from build123d import *

# Parameters (mm, degrees)
F1_DEPTH = 30.1625
F2_R     = 3.175
F3_DEPTH = 19.051
F4_R     = 3.175
F5_DEPTH = 19.051


with BuildPart() as f1:
    # F0 (on Front) → F1 (new body)
    with BuildSketch(Plane.XZ):
        with BuildLine():
            ThreePointArc((9.525, 7.9375), (9.060032, 9.060032), (7.9375, 9.525))
            Line((7.9375, 9.525), (-7.9375, 9.525))
            ThreePointArc((-7.9375, 9.525), (-9.060032, 9.060032), (-9.525, 7.9375))
            Line((-9.525, 7.9375), (-9.525, -7.9375))
            ThreePointArc((-9.525, -7.9375), (-9.060032, -9.060032), (-7.9375, -9.525))
            Line((-7.9375, -9.525), (7.9375, -9.525))
            ThreePointArc((7.9375, -9.525), (9.060032, -9.060032), (9.525, -7.9375))
            Line((9.525, -7.9375), (9.525, 7.9375))
        make_face()
    extrude(amount=F1_DEPTH)

    # F2 (on face) → F3 (cut, through all)
    with BuildSketch(Plane.XY.offset(9.525)):
        with Locations((0, -23.8125)):
            Circle(F2_R)
    extrude(amount=-F3_DEPTH, mode=Mode.SUBTRACT)

    # F4 (on face) → F5 (cut, through all)
    with BuildSketch(Plane(origin=(-9.525, 0, 0), x_dir=(0, -1, 0), z_dir=(-1, 0, 0))):
        with Locations((6.35, 0)):
            Circle(F4_R)
    extrude(amount=-F5_DEPTH, mode=Mode.SUBTRACT)


solid = f1.part
Geometry: final body of the model. Coordinates: model frame, mm. Coordinates: 2 decimals unless noted, no trailing zeros. Order: outer loops, then holes, each group sorted by start corner. A loop starts at its lowest first (then second) coordinate and runs counter-clockwise, first axis right, second up.
(1) Draft query along X for faces 1 (the face through (-9.05, -14.87, 9.07)), 2 (the face through (1.465, -26.629, 0.133)), 3 (the face through (9.525, -15, 0)). Return one class per face: pulls with the +X half, pulls with the -X half, needs draft (parallel to the pull), parting line crosses it, or undercut.
(2) Section query B-B (x = 0). State how many separate pieces and enclosed holes the cut face has, plus the area to 3 significant figures.
(3) Section query A-A (y = -6.35). Return the cut outline in (x, z) (1 decimal).
(4) Material intervals for probe 1 along Y at (x, z) = (0, 4); probe 2 along Z at (x, y) = (1.5, -6.35) (3 decimals); probe 3 along Y at (x, z) = (0, 1), sorted ascending.
(5) First-contact query: pin 1 (4 mm diameter, centred on x = 0, y = -23.81, fed in from +Z). Flat tip, straight axial feed; report the tip coordinate or a pass-through.
Solution:
1. face 1: pulls with the -X half
1. face 2: undercut
1. face 3: pulls with the +X half
2. separate pieces: 2
2. enclosed holes: 1
2. area: 422 mm2
3. outline: (-9.5, -7.9) arc R1.6 ccw to (-7.9, -9.5) - (7.9, -9.5) arc R1.6 ccw to (9.5, -7.9) - (9.5, -3.2) - (-9.5, -3.2) - close; (-9.5, 3.2) - (9.5, 3.2) - (9.5, 7.9) arc R1.6 ccw to (7.9, 9.5) - (-7.9, 9.5) arc R1.6 ccw to (-9.5, 7.9) - close
4. probe 1: y = -30.16 to -26.99, -20.64 to 0
4. probe 2: z = -9.525 to -3.175, 3.175 to 9.525
4. probe 3: y = -30.16 to -26.99, -20.64 to -9.36, -3.34 to 0
5. pin 1: passes through
